For this review, use the dimensioned drawing (mm, ordinates from the lowest corner) and the shaded views. A direction names the side the tool comes from. Coordinates: 2 decimals unless noted, no trailing zeros. Write each loop counter-clockwise with the first axis right and the second up, starting at its lowest first coordinate (ties: lowest second). Pieces come first, ordered by that corner, then holes. Notation, with made-up numbers: (71.25, 33) - (79.25, 33) arc R17 cw to (79.25, 52) - close; hole circle Ø2 at (57.25, 46.25). An arc over 180 degrees is marked (long way). Put each result on its own line as item: value.
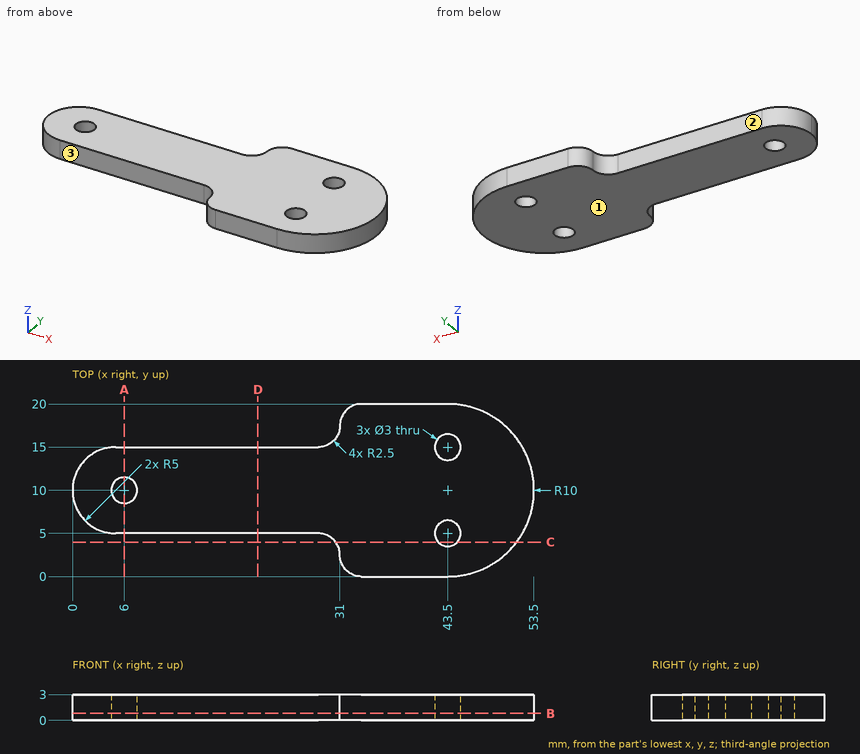
1. Machinability: for the marked faces 1, 2 and 3, which of the approach directions +Z, -Z, +X, -X, +Y, -Y give a long, thin tool a straight path to every point of the face, cutting with its end or side? Answer none if there is none.
Determined:
face 1: -Z, +X, -X, +Y, -Y
face 2: +Z, -Z, -X, +Y
face 3: +Z, -Z, -X, -Y
2. For pin 1 Ø1 at (y, z) = (8, 1) entering from -X; pin 2 Ø1 at (x, z) = (7, 0.5) entering from -Y; pin 3 Ø1.5 at (y, z) = (3, 0.5) entering from -X (3 decimals); pin 4 Ø1.8 at (x, y) = (43.5, 5) entering from -Z, all flat-tipped, find the tip position at first contact; note any pin that passes through.
Determined:
pin 1: stops at x = 0.23
pin 2: stops at y = 5
pin 3: stops at x = 30.665
pin 4: passes through
3. Consider section B-B on z = 0.8. Give the number of separate pieces and of enclosed holes in the cut face, plus the area to 3 significant figures.
Determined:
separate pieces: 1
enclosed holes: 3
area: 685 mm^2
4. Consider section D-D on x = 21.5. State the section outline as (y, z) points, plus the area to 3 significant figures.
Determined:
outline: (5, 0) - (15, 0) - (15, 3) - (5, 3) - close
area: 30.0 mm^2
5. Consider section A-A on x = 6. State the section outline as (y, z) points, plus the area to 3 significant figures.
Determined:
outline: (5, 0) - (8.5, 0) - (8.5, 3) - (5, 3) - close; (11.5, 0) - (15, 0) - (15, 3) - (11.5, 3) - close
area: 21.0 mm^2
6. To check wall thickness, follow probe 1 along Y at (x, z) = (43.5, 1.05); probe 2 along Y at (x, z) = (43, 2.6); probe 3 along Y at (x, z) = (25.5, 2.8). State the ranges of each line that lie inside material, in increasing order.
Determined:
probe 1: y = 0 to 3.5, 6.5 to 13.5, 16.5 to 20
probe 2: y = 0 to 3.59, 6.41 to 13.59, 16.41 to 20
probe 3: y = 5 to 15
7. Consider section C-C on y = 4. State the section outline as (x, z) points, plus the area to 3 significant figures.
Determined:
outline: (30.5, 0) - (42.38, 0) - (42.38, 3) - (30.5, 3) - close; (44.62, 0) - (51.5, 0) - (51.5, 3) - (44.62, 3) - close
area: 56.3 mm^2
